Geometry check sheet. Reference: the model listing, model coordinates, mm. Coordinates: 2 decimals unless noted, no trailing zeros. Loops run counter-clockwise (first coordinate to the right, second up) from the corner with the lowest first, then second, coordinate; pieces in that order, holes last. Notation, with made-up numbers: (83.25, 77.5) - (116.25, 77.5) arc R26 cw to (116.25, 98.5) - close; hole circle Ø4 at (55, 53). An arc over 180 degrees is marked (long way). Write item = value, one per line. Start each with the question number.
from build123d import *

# Parameters (mm, degrees)
SKETCH_3_R          = 8
EXTRUDE_1_DEPTH     = 5
SKETCH_4_R          = 4
CUT_EXTRUDE_1_DEPTH = 213.248558243
SKETCH_5_R          = 1
EXTRUDE_3_DEPTH     = 5


with BuildPart() as part:
    # 草图3 → 凸台-拉伸1 (new body)
    with BuildSketch(Plane.XY):
        with BuildLine():
            ThreePointArc((203.259167971, -8.750002099), (194.509167971, -2.099e-06), (203.259167971, 8.749997901))
            Line((203.259167971, 8.749997901), (0, 8.749997901))
            Line((0, 8.749997901), (-11.740832029, 8))
            ThreePointArc((-11.740832029, 8), (-6.08397778, 5.656854249), (-3.740832029, 0))
            ThreePointArc((-3.740832029, 0), (-6.08397778, -5.656854249), (-11.740832029, -8))
            Line((-11.740832029, -8), (0, -8.750038444))
            Line((0, -8.750038444), (203.259167971, -8.750002099))
        make_face()
        with Locations((-11.740832029, 0)):
            Circle(SKETCH_3_R)
        with BuildLine():
            ThreePointArc((212.009167971, -2.099e-06), (209.446352306, 6.187182236), (203.259167971, 8.749997901))
            Line((203.259167971, 8.749997901), (203.259167971, -8.750002099))
            ThreePointArc((203.259167971, -8.750002099), (209.446352306, -6.187186435), (212.009167971, -2.099e-06))
        make_face()
        with BuildLine():
            Line((203.259167971, -8.750002099), (203.259167971, 8.749997901))
            ThreePointArc((203.259167971, 8.749997901), (194.509167971, -2.099e-06), (203.259167971, -8.750002099))
        make_face()
    extrude(amount=EXTRUDE_1_DEPTH)

    # 草图4 → 切除-拉伸1 (cut, through all)
    with BuildSketch(Plane.XY.offset(5)):
        with Locations((-11.740832029, 0)):
            Circle(SKETCH_4_R)
        with Locations((203.259167971, -2.099e-06)):
            Circle(SKETCH_4_R)
    extrude(amount=-CUT_EXTRUDE_1_DEPTH, mode=Mode.SUBTRACT)

    # 草图5 → 凸台-拉伸3 (add)
    with BuildSketch(Plane.XY):
        with BuildLine():
            ThreePointArc((-11.740832029, -8), (-19.131223835, -3.063022848), (-17.400066767, 5.654472759))
            Line((-17.400066767, 5.654472759), (-31.381865156, -8.327324627))
            ThreePointArc((-31.381865156, -8.327324627), (-31.320161123, -19.702071726), (-19.94675289, -19.516966077))
            Line((-19.94675289, -19.516966077), (-9.081705309, -8.169872737))
            Line((-9.081705309, -8.169872737), (-11.740832029, -8))
        make_face()
        with Locations((-28.81851625, -10.634029839)):
            Circle(SKETCH_5_R, mode=Mode.SUBTRACT)
        with Locations((-22.374861868, -17.077684221)):
            Circle(SKETCH_5_R, mode=Mode.SUBTRACT)
    extrude(amount=EXTRUDE_3_DEPTH)


solid = part.part
(1) Scan lines: line 1 (X direction, y = -3, z = 2.7); line 2 (Y direction, x = 0, z = 0.7); line 3 (X direction, y = -2, z = 2.65). Record each from-to range of solid material in increasing order.
(2) Depth check by flat-ended pin: pin 1 (3 mm diameter, centred on x = 11.5, y = -10, fed in from +Z). Enter the tip coordinate at first touch or a pass-through.
(3) Sectioned sample at B-B on x = 102.5. Enter the section's corners in (y, z), plus the area to 3 significant figures.
(4) Sectioned sample at A-A on z = 2. Enter the section's corners in (x, y), plus the area to 3 significant figures.
(5) Draft check along X on faces 1 (the face through (-31, -20, 2)), 2 (the face through (-24.293, -1.239, 2.465)), 3 (the face through (100, -8.75, 2)), 4 (the face through (-4.604, -8.456, 2.465)). Enter one of: pulls with the +X half, pulls with the -X half, needs draft (parallel to the pull), parting line crosses it, or undercut.
Working result:
q1.line_1 = -26.05 to -14.39, -9.1 to 200.61, 205.9 to 211.48
q1.line_2 = -8.75 to 8.75
q1.line_3 = -25.05 to -15.2, -8.28 to 199.8, 206.72 to 211.78
q2.pin_1 = 5
q3.outline = (-8.75, 0) - (8.75, 0) - (8.75, 5) - (-8.75, 5) - close
q3.area = 87.5 mm2
q4.outline = (-31.38, -8.33) arc R8 ccw (long way) to (-19.95, -19.52) - (-9.08, -8.17) - (0, -8.75) - (203.26, -8.75) arc R8.75 ccw to (203.26, 8.75) - (0, 8.75) - (-11.74, 8) arc R8 ccw to (-17.4, 5.65) - close; hole circle Ø2 at (-28.82, -10.63); hole circle Ø2 at (-22.37, -17.08); hole circle Ø8 at (-11.74, 0); hole circle Ø8 at (203.26, 0)
q4.area = 4,180 mm2
q5.face_1 = parting line crosses it
q5.face_2 = pulls with the -X half
q5.face_3 = needs draft
q5.face_4 = undercut
